Work out the finished part from the listing and answer in its coordinate system (mm). Coordinates: 2 decimals unless noted, no trailing zeros. Order: outer loops, then holes, each group sorted by start corner. A loop starts at its lowest first (then second) coordinate and runs counter-clockwise, first axis right, second up.
1. The part is cut by section C-C, the plane z = 5. Give the vertices of the cut face in (x, y) (3 decimals).
2. Flat-ended cylindrical pins translate along their axes: pin 1 Ø5 at (y, z) = (9.525, 22.098) entering from -X; pin 2 Ø2.5 at (y, z) = (0, -30.16) entering from -X; pin 3 Ø1 at (x, z) = (2, -26) entering from -Y. Find the tip coordinate at first contact, or state that the pin passes through.
3. The part is cut by section A-A, the plane z = 11. Give the vertices of the cut face in (x, y) (3 decimals), then the cut area to 3 significant figures.
4. The part is cut by section B-B, the plane y = 0. Count the separate pieces of the cut face and the enclosed holes in it, then the cut area to 3 significant figures.
5. Find the intervals of material crossed by probe 1 along Y at (x, z) = (1, 4); probe 2 along Z at (x, y) = (0.7, 2.5); probe 3 along Z at (x, y) = (1.1, 1.5), in increasing order.
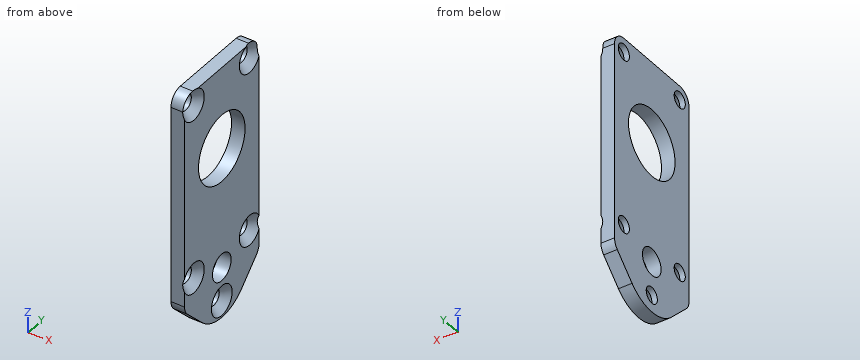
Autodesk Inventor part; units mm, degrees
ref_plane "YZ Plane" through (0, 0, 0) normal (1, 0, 0) x (0, 1, 0)
ref_plane "XZ Plane" through (0, 0, 0) normal (0, 1, 0) x (-1, 0, 0)
ref_plane "XY Plane" through (0, 0, 0) normal (0, 0, 1) x (1, 0, 0)
sketch "Sketch1" plane through (0, 0, 0) normal (1, 0, 0) x (0, 1, 0)
  line L0 (-12.7, 25.4) -> (12.7, 25.4)
  line L1 (12.7, 25.4) -> (12.7, -25.4)
  line L2 (12.7, -25.4) -> (-12.7, -25.4) construction
  line L3 (-12.7, -25.4) -> (-12.7, 25.4)
  line L4 (-12.7, 25.4) -> (12.7, -25.4) construction
  line L5 (12.7, 25.4) -> (-12.7, -25.4) construction
  line L6 (0, 25.4) -> (0, -25.4) construction
  circle A0 centre (0, -22.225) radius 3.175
  line L7 (-3.175, -15.875) -> (3.175, -15.875) construction
  line L8 (3.175, -15.875) -> (3.175, -34.925) construction
  line L9 (3.175, -34.925) -> (-3.175, -34.925)
  line L10 (-3.175, -34.925) -> (-3.175, -15.875) construction
  line L11 (-3.175, -15.875) -> (3.175, -34.925) construction
  line L12 (3.175, -15.875) -> (-3.175, -34.925) construction
  line L13 (12.7, -25.4) -> (3.175, -34.925)
  line L14 (-3.175, -34.925) -> (-12.7, -25.4)
  circle A1 centre (0, 6.175) radius 7.9375
  point P0 (0, 0)
  dimension "d0" = 25.4
  dimension "d1" = 50.8
  dimension "d2" = 6.35
  dimension "d4" = 6.35
  dimension "d5" = 9.525
  dimension "d6" = 15.875
  dimension "d7" = 28.4
extrude "Extrusion1" add sketch "Sketch1" along normal blind 3.175
fillet "Fillet1" radius 9.525 2 edges at (1.5875, 3.175, -34.925) (1.5875, -3.175, -34.925)
fillet "Fillet2" radius 3.175 4 edges at (1.5875, 12.7, 25.4) (1.5875, -12.7, 25.4) (1.5875, 12.7, -25.4) (1.5875, -12.7, -25.4)
sketch "Sketch2" plane through (3.175, 0, 0) normal (1, 0, 0) x (0, 0, -1)
  point P0 (19.05, 9.525)
  point P1 (30.1625, 0)
  point P2 (19.05, -9.525)
  point P3 (-22.098, 9.525)
  point P4 (-22.098, -9.525)
hole "Hole1" at (3.175, 9.525, -19.05) at (3.175, 0, -30.1625) at (3.175, -9.525, -19.05) at (3.175, 9.525, 22.098) at (3.175, -9.525, 22.098) direction (-1, 0, 0) diameter 3.7973 end through all countersink diameter 7.0866 countersink angle 82
properties part number "Face PLate" material "UHMW, White"
Geometry says:
1. outline: (0, -12.7) - (3.175, -12.7) - (3.175, -7.85) - (0, -7.85) - close; (0, 7.85) - (3.175, 7.85) - (3.175, 12.7) - (0, 12.7) - close
2. pin 1: stops at x = 0
2. pin 2: passes through
2. pin 3: stops at y = -12.37
3. outline: (0, -12.7) - (3.175, -12.7) - (3.175, -6.303) - (0, -6.303) - close; (0, 6.303) - (3.175, 6.303) - (3.175, 12.7) - (0, 12.7) - close
3. area: 40.6 mm2
4. separate pieces: 4
4. enclosed holes: 0
4. area: 103 mm2
5. probe 1: y = -12.7 to -7.63, 7.63 to 12.7
5. probe 2: z = -33.82 to -24.18, -20.27 to -1.36, 13.71 to 25.4
5. probe 3: z = -34.04 to -31.33, -29 to -25.02, -19.43 to -1.62, 13.97 to 25.4
